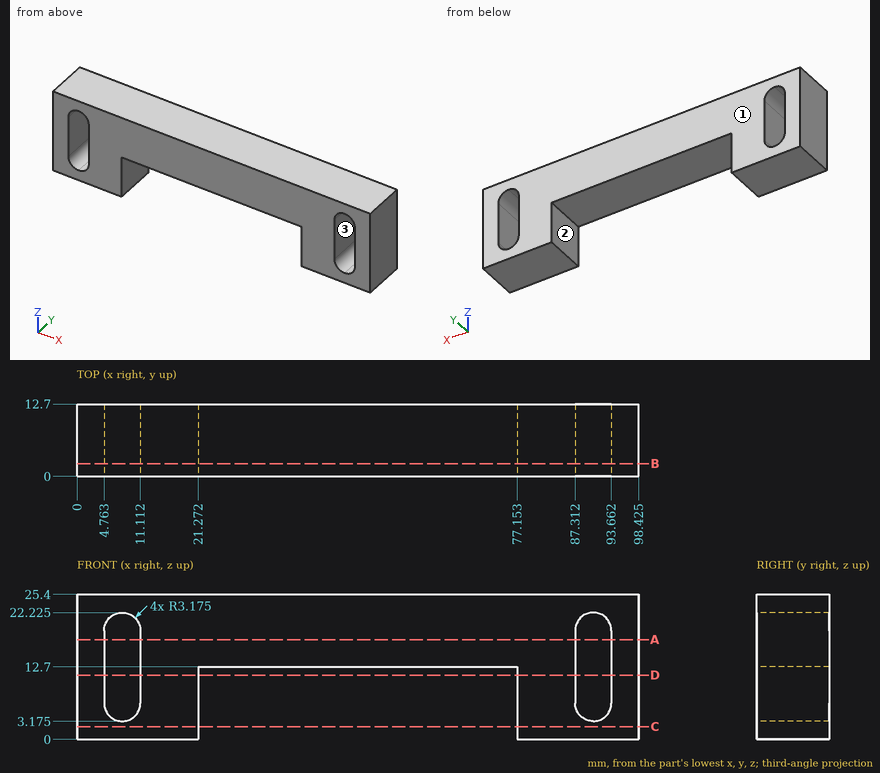
Can you work these out from the drawing? Everything is in mm from the part's minimum corner. A direction names the side the tool comes from. Give positions to 0.01 mm unless a question says otherwise; leave off trailing zeros. Loops run counter-clockwise (first coordinate to the right, second up) from the corner with the lowest first, then second, coordinate; pieces in that order, holes last. Notation, with made-up numbers: (28.25, 29) -> (62.25, 29) arc R31 cw to (62.25, 67) -> close; hole circle Ø11 at (75, -29.75). An arc over 180 degrees is marked (long way). Put each result on its own line as item: value.
(1) For the marked faces 1, 2 and 3, which set-ups out of +Z, -Z, +X, -X, +Y, -Y let a thin tool reach every point of the face, with its end or its side?
Computed:
face 1: +Z, -Z, +X, -X, +Y
face 2: -Z, +Y, -Y
face 3: +Y, -Y
(2) Imagine slicing it at A-A on z = 17.5. Write out the boundary of the cut face in (x, y) (1 decimal).
Computed:
outline: (0, 0) -> (4.8, 0) -> (4.8, 12.7) -> (0, 12.7) -> close; (11.1, 0) -> (87.3, 0) -> (87.3, 12.7) -> (11.1, 12.7) -> close; (93.7, 0) -> (98.4, 0) -> (98.4, 12.7) -> (93.7, 12.7) -> close
(3) Imagine slicing it at C-C on z = 2.25. Write out the boundary of the cut face in (x, y) (1 decimal), plus the area to 3 significant figures.
Computed:
outline: (0, 0) -> (21.3, 0) -> (21.3, 12.7) -> (0, 12.7) -> close; (77.2, 0) -> (98.4, 0) -> (98.4, 12.7) -> (77.2, 12.7) -> close
area: 540 mm^2
(4) Please list where these lines run through material, in increasing order: probe 1 along X at (y, z) = (8, 18) (1 decimal); probe 2 along X at (y, z) = (10, 6) (1 decimal); probe 3 along X at (y, z) = (9, 12.5) (1 decimal). Write a range as [from, to].
Computed:
probe 1: [0, 4.8], [11.1, 87.3], [93.7, 98.4]
probe 2: [0, 4.8], [11.1, 21.3], [77.2, 87.3], [93.6, 98.4]
probe 3: [0, 4.8], [11.1, 21.3], [77.2, 87.3], [93.7, 98.4]
(5) Imagine slicing it at D-D on z = 11.25. Write out the boundary of the cut face in (x, y) (1 decimal), plus the area to 3 significant figures.
Computed:
outline: (0, 0) -> (4.8, 0) -> (4.8, 12.7) -> (0, 12.7) -> close; (11.1, 0) -> (21.3, 0) -> (21.3, 12.7) -> (11.1, 12.7) -> close; (77.2, 0) -> (87.3, 0) -> (87.3, 12.7) -> (77.2, 12.7) -> close; (93.7, 0) -> (98.4, 0) -> (98.4, 12.7) -> (93.7, 12.7) -> close
area: 379 mm^2
(6) Imagine slicing it at B-B on y = 2.25. State how many separate pieces and enclosed holes the cut face has, plus the area to 3 significant figures.
Computed:
separate pieces: 1
enclosed holes: 2
area: 1,570 mm^2
